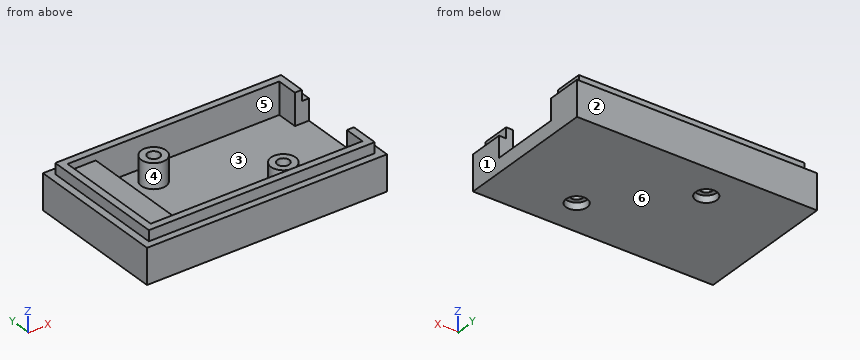
from build123d import *

# Parameters (mm, degrees)
SKETCH_1_W          = 34
SKETCH_1_H          = 20
EXTRUDE_1_DEPTH     = 6.5
SKETCH_2_W          = 30
SKETCH_2_H          = 16
CUT_EXTRUDE_1_DEPTH = 4.5
SKETCH_3_W          = 4.5
SKETCH_3_H          = 10
CUT_EXTRUDE_2_DEPTH = 2
CUT_EXTRUDE_3_DEPTH = 1.5
SKETCH_5_W          = 4
SKETCH_5_H          = 16
EXTRUDE_2_DEPTH     = 3.5
SKETCH_6_R          = 1.75
EXTRUDE_3_DEPTH     = 3.5
SKETCH_7_R          = 0.85
CUT_EXTRUDE_4_DEPTH = 21.475595229
SKETCH_8_R          = 1.5
CUT_EXTRUDE_5_DEPTH = 1


with BuildPart() as part:
    # 草图1 → 凸台-拉伸1 (new body)
    with BuildSketch(Plane.XY):
        Rectangle(SKETCH_1_W, SKETCH_1_H)
    extrude(amount=EXTRUDE_1_DEPTH)

    # 草图2 → 切除-拉伸1 (cut)
    with BuildSketch(Plane.XY.offset(6.5)):
        Rectangle(SKETCH_2_W, SKETCH_2_H)
    extrude(amount=-CUT_EXTRUDE_1_DEPTH, mode=Mode.SUBTRACT)

    # 草图3 → 切除-拉伸2 (cut)
    with BuildSketch(Plane(origin=(17, 0, 0), x_dir=(0, 0, -1), z_dir=(1, 0, 0))):
        with Locations((-4.25, 0)):
            Rectangle(SKETCH_3_W, SKETCH_3_H)
    extrude(amount=-CUT_EXTRUDE_2_DEPTH, mode=Mode.SUBTRACT)

    # 草图4 → 切除-拉伸3 (cut)
    with BuildSketch(Plane.XY.offset(6.5)):
        Polygon((16, 5), (16, 9), (-16, 9), (-16, -9), (16, -9), (16, -5), (17, -5), (17, -10), (-17, -10), (-17, 10), (17, 10), (17, 5), align=None)
    extrude(amount=-CUT_EXTRUDE_3_DEPTH, mode=Mode.SUBTRACT)

    # 草图5 → 凸台-拉伸2 (add)
    with BuildSketch(Plane.XY.offset(2)):
        with Locations((-13, 0)):
            Rectangle(SKETCH_5_W, SKETCH_5_H)
    extrude(amount=EXTRUDE_2_DEPTH)

    # 草图6 → 凸台-拉伸3 (add)
    with BuildSketch(Plane.XY.offset(2)):
        with Locations((-5, 5)):
            Circle(SKETCH_6_R)
        with Locations((6, -5)):
            Circle(SKETCH_6_R)
    extrude(amount=EXTRUDE_3_DEPTH)

    # 草图7 → 切除-拉伸4 (cut, through all)
    with BuildSketch(Plane.XY.offset(5.5)):
        with Locations((-5, 5)):
            Circle(SKETCH_7_R)
        with Locations((6, -5)):
            Circle(SKETCH_7_R)
    extrude(amount=-CUT_EXTRUDE_4_DEPTH, mode=Mode.SUBTRACT)

    # 草图8 → 切除-拉伸5 (cut)
    with BuildSketch(Plane(origin=(0, 0, 0), x_dir=(-1, 0, 0), z_dir=(0, 0, -1))):
        with Locations((-6, -5)):
            Circle(SKETCH_8_R)
        with Locations((5, 5)):
            Circle(SKETCH_8_R)
    extrude(amount=-CUT_EXTRUDE_5_DEPTH, mode=Mode.SUBTRACT)


solid = part.part
For this review, take the finished solid that the model builds, in its own axes (mm). Face numbers are marked on the shaded views. A direction names the side the tool comes from. Round coordinates to 2 decimals unless told otherwise and drop trailing zeros. Loops run counter-clockwise (first coordinate to the right, second up) from the corner with the lowest first, then second, coordinate; pieces in that order, holes last. Notation, with made-up numbers: (59.5, 18) - (68.5, 18) arc R16 ccw to (68.5, 22) - close; hole circle Ø10 at (-25.75, 80). An arc over 180 degrees is marked (long way). Answer as CSV lines item,"result".
(1) Wall thickness on line 1 (Y direction, x = 6, z = 2.4); line 2 (Y direction, x = 5.5, z = 4.5); line 3 (Y direction, x = -10.5, z = 2.75): over which ranges is each line inside the solid? List them lowest first.
Checked values:
line 1,"y = -10 to -8, -6.75 to -5.85, -4.15 to -3.25, 8 to 10"
line 2,"y = -10 to -8, -6.68 to -5.69, -4.31 to -3.32, 8 to 10"
line 3,"y = -10 to -8, 8 to 10"
(2) Consider section D-D on z = 0.5. Give the boundary of the cut face in (x, y), then the cut area to 3 significant figures.
Checked values:
outline,"(-17, -10) - (17, -10) - (17, 10) - (-17, 10) - close; hole circle Ø3 at (-5, 5); hole circle Ø3 at (6, -5)"
area,"666 mm2"
(3) Consider section A-A on z = 2.75. Give the boundary of the cut face in (x, y).
Checked values:
outline,"(-17, -10) - (17, -10) - (17, -5) - (15, -5) - (15, -8) - (-11, -8) - (-11, 8) - (15, 8) - (15, 5) - (17, 5) - (17, 10) - (-17, 10) - close; circle Ø3.5 at (-5, 5); circle Ø3.5 at (6, -5); hole circle Ø1.7 at (-5, 5); hole circle Ø1.7 at (6, -5)"
(4) Mouldability with a two-part tool opening along X and no side actions: class the marked faces 1, 2, 3 and 4 as +X half, -X half, draft (parallel to the pull), parting line (faces both ways), or undercut.
Checked values:
face 1,"+X half"
face 2,"draft"
face 3,"undercut"
face 4,"undercut"
(5) Tool access review of the marked faces 5 and 6: name each direction out of +Z, -Z, +X, -X, +Y, -Y from which nothing blocks a thin tool from reaching the whole face with its end or side.
Checked values:
face 5,"+Z"
face 6,"-Z, +X, -X, +Y, -Y"
(6) Insertion check: P1, Ø1, axis at x = -10, y = 6.5, coming from the +Z side; P2, Ø1.8, axis at x = -5, y = 4.5, coming from the +Z side; P3, Ø1.5, axis at x = 6, y = -5, coming from the -Z side; P4, Ø2.5, axis at x = -5, y = 5, coming from the -Z side. Each pin has a flat end and moves straight along its axis. Give the tip position at first contact, or say it passes through.
Checked values:
P1,"stops at z = 2"
P2,"stops at z = 5.5"
P3,"passes through"
P4,"stops at z = 1"
(7) Consider section B-B on x = 6. Give the boundary of the cut face in (y, z), then the cut area to 3 significant figures.
Checked values:
outline,"(-10, 0) - (-6.5, 0) - (-6.5, 1) - (-5.85, 1) - (-5.85, 5.5) - (-6.75, 5.5) - (-6.75, 2) - (-8, 2) - (-8, 6.5) - (-9, 6.5) - (-9, 5) - (-10, 5) - close; (-4.15, 1) - (-3.5, 1) - (-3.5, 0) - (10, 0) - (10, 5) - (9, 5) - (9, 6.5) - (8, 6.5) - (8, 2) - (-3.25, 2) - (-3.25, 5.5) - (-4.15, 5.5) - close"
area,"56.6 mm2"
(8) Consider section C-C on y = 7.5. Give the boundary of the cut face in (x, z), then the cut area to 3 significant figures.
Checked values:
outline,"(-17, 0) - (17, 0) - (17, 5) - (16, 5) - (16, 6.5) - (15, 6.5) - (15, 2) - (-11, 2) - (-11, 5.5) - (-15, 5.5) - (-15, 6.5) - (-16, 6.5) - (-16, 5) - (-17, 5) - close"
area,"97.0 mm2"
